from build123d import *

# Parameters (mm, degrees)
F0_W     = 12.7
F0_H     = 19.8
F1_DEPTH = 12
F0_R     = 2.75
F2_DEPTH = 2
F3_R     = 0.6
F4_R     = 0.6


# Not quite as in the source:
# - a feature names something its author has since deleted; it is built from what else it names


with BuildPart() as f1:
    # F0 (on Top) → F1 (new body)
    with BuildSketch(Plane.XY):
        with Locations((13.45, 9.9)):
            Rectangle(F0_W, F0_H)
        Polygon((17.8, 14.6), (17.8, 2), (9.6, 2), (9.6, 14.6), (12.3, 17.8), (15.1, 17.8), align=None, mode=Mode.SUBTRACT)
    extrude(amount=F1_DEPTH)

    # F0 (on Top) → F2 (join)
    with BuildSketch(Plane.XY):
        Polygon((9.6, 2), (17.8, 2), (17.8, 14.6), (15.1, 17.8), (12.3, 17.8), (9.6, 14.6), align=None)
        with Locations((13.7, 6.1)):
            Circle(F0_R, mode=Mode.SUBTRACT)
        with Locations((13.7, 13.1)):
            Circle(F0_R, mode=Mode.SUBTRACT)
    extrude(amount=F2_DEPTH)

    # F3
    f3_edges = [f1.edges().sort_by_distance(p)[0] for p in [
        (13.45, 0, 12),
        (19.8, 9.9, 12),
        (13.45, 19.8, 12),
    ]]
    fillet(f3_edges, radius=F3_R)

    # F4
    f4_edges = [f1.edges().sort_by_distance(p)[0] for p in [
        (13.45, 0, 0),
        (19.8, 9.9, 0),
        (13.45, 19.8, 0),
    ]]
    fillet(f4_edges, radius=F4_R)


solid = f1.part
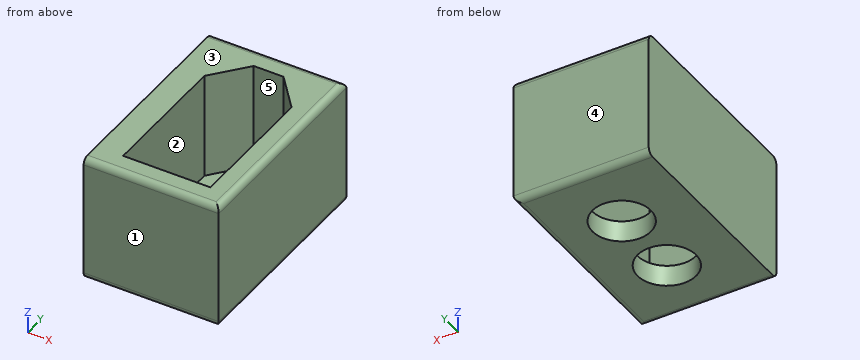
For this review, take the finished solid that the model builds, in its own axes (mm). Face numbers are marked on the shaded views. A direction names the side the tool comes from. Give positions to 0.01 mm unless a question says otherwise; leave off trailing zeros. Loops run counter-clockwise (first coordinate to the right, second up) from the corner with the lowest first, then second, coordinate; pieces in that order, holes last.
Item 1: Take a section at C-C, the plane z = 10.5. State the section outline as (x, y) points.
Item 2: Insertion check: pin 1 (3.5 mm diameter, centred on x = 13.7, y = 13.1, fed in from +Z); pin 2 (6.5 mm diameter, centred on x = 13.5, y = 8.5, fed in from +Z). Each pin has a flat end and moves straight along its axis. Give the tip position at first contact, or say it passes through.
Item 3: Tool access review of the marked faces 4 and 5: name each direction out of +Z, -Z, +X, -X, +Y, -Y from which nothing blocks a thin tool from reaching the whole face with its end or side.
Item 4: Take a section at A-A, the plane y = 6.1. State the section outline as (x, z) points.
Item 5: For line 1 along Y through (x, z) = (13.7, 1.2); line 2 along X through (y, z) = (6, 4.25); line 3 along Y through (x, z) = (11.75, 0.5), list the stretches that pass through material, from the lowest coordinate up.
Item 6: Draft analysis for pull direction Y (two halves, no side actions). For the marked faces 1, 2 and 3, state which applies: +Y half, -Y half, draft (parallel to the pull), parting line (faces both ways), or undercut.
Item 7: Take a section at D-D, the plane z = 1. State the section outline as (x, y) points.
Item 8: Take a section at B-B, the plane x = 13.7. State the section outline as (y, z) points, and give its area (3 significant figures).
Calculated:
1. outline: (7.1, 0) - (19.8, 0) - (19.8, 19.8) - (7.1, 19.8) - close; hole (9.6, 2) - (17.8, 2) - (17.8, 14.6) - (15.1, 17.8) - (12.3, 17.8) - (9.6, 14.6) - close
2. pin 1: passes through
2. pin 2: stops at z = 2
3. face 4: +Z, -Z, +X, -X, +Y
3. face 5: +Z
4. outline: (7.1, 0) - (10.95, 0) - (10.95, 2) - (9.6, 2) - (9.6, 12) - (7.1, 12) - close; (16.45, 0) - (19.2, 0) arc R0.6 ccw to (19.8, 0.6) - (19.8, 11.4) arc R0.6 ccw to (19.2, 12) - (17.8, 12) - (17.8, 2) - (16.45, 2) - close
5. line 1: y = 0 to 3.35, 8.85 to 10.35, 15.85 to 19.8
5. line 2: x = 7.1 to 9.6, 17.8 to 19.8
5. line 3: y = 0.01 to 4.16, 8.04 to 11.16, 15.04 to 19.79
6. face 1: -Y half
6. face 2: undercut
6. face 3: draft
7. outline: (7.1, 0) - (19.8, 0) - (19.8, 19.8) - (7.1, 19.8) - close; hole circle Ø5.5 at (13.7, 6.1); hole circle Ø5.5 at (13.7, 13.1)
8. outline: (0, 0.6) arc R0.6 ccw to (0.6, 0) - (3.35, 0) - (3.35, 2) - (2, 2) - (2, 12) - (0.6, 12) arc R0.6 ccw to (0, 11.4) - close; (8.85, 0) - (10.35, 0) - (10.35, 2) - (8.85, 2) - close; (15.85, 0) - (19.2, 0) arc R0.6 ccw to (19.8, 0.6) - (19.8, 11.4) arc R0.6 ccw to (19.2, 12) - (17.8, 12) - (17.8, 2) - (15.85, 2) - close
8. area: 57.3 mm2
